Verification items for this drawing (mm, ordinates from the low corner). A direction names the side the tool comes from. Round coordinates to 2 decimals unless told otherwise and drop trailing zeros. Loops run counter-clockwise (first coordinate to the right, second up) from the corner with the lowest first, then second, coordinate; pieces in that order, holes last. Notation, with made-up numbers: M 52,66.25 L 66,66.25 A10 ccw 66,81.25 Z; hole C 37,-22 d8. An arc over 180 degrees is marked long. Use one line per item in the form item = value. Start each with the question number.
1. Go/stop test with flat-tipped pins: pin 1 (1.8 mm diameter, centred on y = 14, z = 30.5, fed in from +X); pin 2 (5 mm diameter, centred on y = 9.5, z = 54.5, fed in from -X); pin 3 (8 mm diameter, centred on y = 10, z = 54, fed in from +X). Record where each tip stops, or that it passes through.
2. Cross-section at C-C (x = 30). Record the boundary of the cut face in (y, z).
3. Set-up check for the marked faces 1, 2 and 3: record each of +Z, -Z, +X, -X, +Y, -Y from which the full face is reachable in a straight line by a thin tool's end or side.
4. Material ranges on line 1 (Y direction, x = 24.4, z = 30); line 2 (Y direction, x = 34, z = 18); line 3 (X direction, y = 13, z = 53.5), recorded low to high.
5. Cross-section at A-A (y = 3.75). Record the boundary of the cut face in (x, z), then the cut area to 3 significant figures.
6. Cross-section at B-B (z = 30). State how many separate pieces and enclosed holes the cut face has, then the cut area to 3 significant figures.
7. Draft check along Z on the marked faces 4 and 5. Enter one of: pulls with the +Z half, pulls with the -Z half, needs draft (parallel to the pull), parting line crosses it, or undercut.
8. Cross-section at D-D (z = 55). Record the boundary of the cut face in (x, y), then the cut area to 4 significant figures.
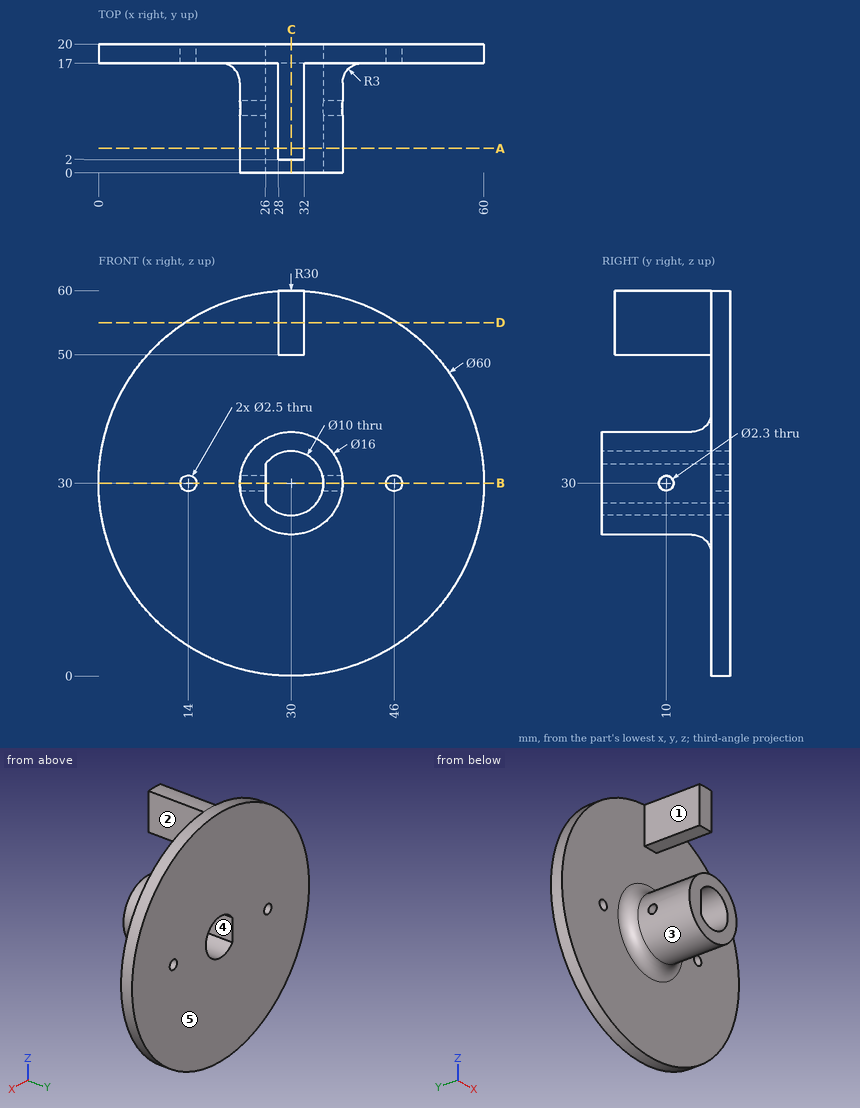
Reported:
q1.pin_1 = 38.13
q1.pin_2 = 28
q1.pin_3 = 32
q2.outline = M 0,22 L 14,22 A3 cw 17,19 L 17,0 L 20,0 L 20,25 L 0,25 Z; M 0,35 L 20,35 L 20,60 L 2,60 L 2,50 L 17,50 L 17,41 A3 cw 14,38 L 0,38 Z
q3.face_1 = +Z, -X, -Y
q3.face_2 = +Z, +X, -Y
q3.face_3 = -Y
q4.line_1 = 0 to 8.85, 11.15 to 20
q4.line_2 = 17 to 20
q4.line_3 = 28 to 32
q5.outline = C 30,30 d16; M 28,50 L 32,50 L 32,59.93 A30 ccw 28,59.93 Z; hole M 26,27 A5 ccw long 26,33 Z
q5.area = 167 mm²
q6.separate_pieces = 6
q6.enclosed_holes = 0
q6.area = 245 mm²
q7.face_4 = undercut
q7.face_5 = needs draft
q8.outline = M 13.42,17 L 28,17 L 28,2 L 32,2 L 32,17 L 46.58,17 L 46.58,20 L 13.42,20 Z
q8.area = 159.5 mm²
